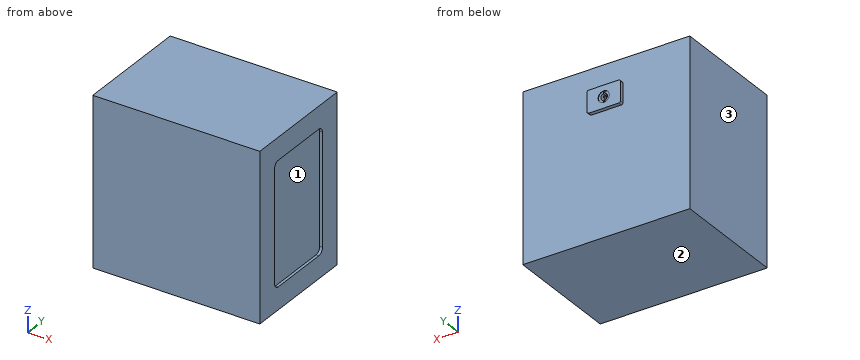
```python
from build123d import *

# Parameters (mm, degrees)
SKETCH1_W           = 300
SKETCH1_H           = 300
BOSS_EXTRUDE1_DEPTH = 210
CUT_EXTRUDE1_DEPTH  = 5
BOSS_EXTRUDE2_DEPTH = 7
SKETCH4_R           = 10
CUT_EXTRUDE2_DEPTH  = 1
SKETCH5_R           = 1.5
CUT_EXTRUDE3_DEPTH  = 10


with BuildPart() as part:
    # Sketch1 → Boss-Extrude1 (new body)
    with BuildSketch(Plane(origin=(0, 0, 0), x_dir=(1, 0, 0), z_dir=(0, 1, 0))):
        Rectangle(SKETCH1_W, SKETCH1_H)
    extrude(amount=BOSS_EXTRUDE1_DEPTH)

    # Sketch2 → Cut-Extrude1 (cut)
    with BuildSketch(Plane(origin=(150, 0, 0), x_dir=(0, 0, -1), z_dir=(1, 0, 0))):
        with BuildLine():
            Line((-100, 170), (100, 170))
            ThreePointArc((100, 170), (107.071067812, 167.071067812), (110, 160))
            Line((110, 160), (110, 50))
            ThreePointArc((110, 50), (107.071067812, 42.928932188), (100, 40))
            Line((100, 40), (-100, 40))
            ThreePointArc((-100, 40), (-107.071067812, 42.928932188), (-110, 50))
            Line((-110, 50), (-110, 160))
            ThreePointArc((-110, 160), (-107.071067812, 167.071067812), (-100, 170))
        make_face()
    extrude(amount=-CUT_EXTRUDE1_DEPTH, mode=Mode.SUBTRACT)

    # Sketch3 → Boss-Extrude2 (add)
    with BuildSketch(Plane(origin=(0, 210, 0), x_dir=(1, 0, 0), z_dir=(0, 1, 0))):
        with BuildLine():
            Line((-27, -110), (27, -110))
            ThreePointArc((27, -110), (29.121320344, -109.121320344), (30, -107))
            Line((30, -107), (30, -73))
            ThreePointArc((30, -73), (29.121320344, -70.878679656), (27, -70))
            Line((27, -70), (-27, -70))
            ThreePointArc((-27, -70), (-29.121320344, -70.878679656), (-30, -73))
            Line((-30, -73), (-30, -107))
            ThreePointArc((-30, -107), (-29.121320344, -109.121320344), (-27, -110))
        make_face()
    extrude(amount=BOSS_EXTRUDE2_DEPTH)

    # Sketch4 → Cut-Extrude2 (cut)
    with BuildSketch(Plane(origin=(0, 217, 0), x_dir=(1, 0, 0), z_dir=(0, 1, 0))):
        with Locations(Location((0, -90, 0), (0, 0, 270))):
            Circle(SKETCH4_R)
    extrude(amount=-CUT_EXTRUDE2_DEPTH, mode=Mode.SUBTRACT)

    # Sketch5 → Cut-Extrude3 (cut)
    with BuildSketch(Plane(origin=(0, 216, 0), x_dir=(1, 0, 0), z_dir=(0, 1, 0))):
        with BuildLine():
            Line((-1.5, -84.190524981), (-1.5, -80.25))
            Line((-1.5, -80.25), (1.5, -80.25))
            Line((1.5, -80.25), (1.5, -84.190524981))
            ThreePointArc((1.5, -84.190524981), (6, -90), (1.5, -95.809475019))
            Line((1.5, -95.809475019), (1.5, -99.75))
            Line((1.5, -99.75), (-1.5, -99.75))
            Line((-1.5, -99.75), (-1.5, -95.809475019))
            ThreePointArc((-1.5, -95.809475019), (-6, -90), (-1.5, -84.190524981))
        make_face()
        with Locations(Location((0, -90, 0), (0, 0, 270))):
            Circle(SKETCH5_R, mode=Mode.SUBTRACT)
    extrude(amount=-CUT_EXTRUDE3_DEPTH, mode=Mode.SUBTRACT)


solid = part.part
```
Check sheet for the modelled part. Datum: model origin and axes. Units: mm. Face numbers are marked on the shaded views. Give positions to 0.01 mm unless a question says otherwise; leave off trailing zeros. Write each loop counter-clockwise with the first axis right and the second up, starting at its lowest first coordinate (ties: lowest second). Pieces come first, ordered by that corner, then holes. Notation, with made-up numbers: (33.5, -37.75) -> (50.5, -37.75) arc R31 ccw to (50.5, -0.75) -> close; hole circle Ø7 at (46.5, 10). An arc over 180 degrees is marked (long way). Use CSV: the item, a comma, the result in double quotes. Start each with the question number.
Q1. Depth check by flat-ended pin: P1, Ø4, axis at x = 41.5, z = 7.5, coming from the +Y side; P2, Ø10, axis at x = -2.5, z = 90, coming from the +Y side; P3, Ø2, axis at y = 214.5, z = 86.5, coming from the +X side. Enter the tip coordinate at first touch or a pass-through.
Q2. Release check for a two-part mould opening along Z. For the marked faces 1, 2 and 3 record: +Z half, -Z half, draft (parallel to the pull), parting line (faces both ways), or undercut.
Q3. Scan lines: line 1 along X through (y, z) = (216.65, 90); line 2 along Y through (x, z) = (127, -12); line 3 along X through (y, z) = (101, -29). Record each from-to range of solid material in increasing order.
Q4. Cross-section at B-B on x = -60.5. Enter the section's corners in (y, z).
Q5. Cross-section at A-A on z = 42.5. Enter the section's corners in (x, y).
Working result:
1,P1,"stops at y = 210"
1,P2,"stops at y = 216"
1,P3,"stops at x = 30"
2,face 1,"undercut"
2,face 2,"-Z half"
2,face 3,"draft"
3,line 1,"x = -30 to -10, 10 to 30"
3,line 2,"y = 0 to 210"
3,line 3,"x = -150 to 145"
4,outline,"(0, -150) -> (210, -150) -> (210, 150) -> (0, 150) -> close"
5,outline,"(-150, 0) -> (150, 0) -> (150, 40) -> (145, 40) -> (145, 170) -> (150, 170) -> (150, 210) -> (-150, 210) -> close"
